Input: part model. Units: mm. Frame: model coordinates. Face numbers are marked on the shaded views. A direction names the side the tool comes from. Coordinates: 2 decimals unless noted, no trailing zeros. Loops run counter-clockwise (first coordinate to the right, second up) from the corner with the lowest first, then second, coordinate; pieces in that order, holes last.
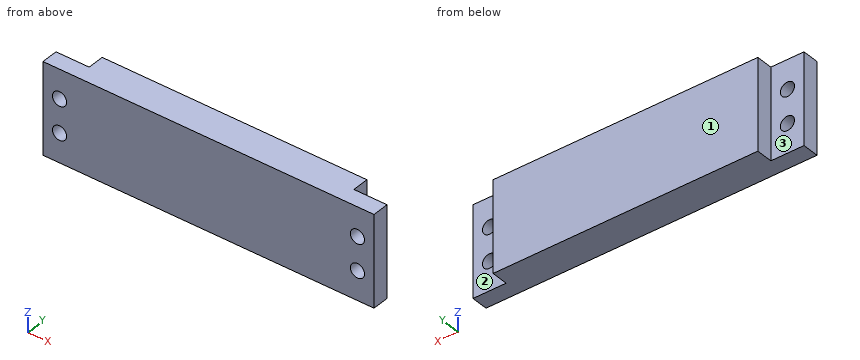
```python
from build123d import *

# Parameters (mm, degrees)
SKETCH1_W           = 63.5
SKETCH1_H           = 17.4625
BOSS_EXTRUDE1_DEPTH = 6.35
SKETCH2_W           = 6.35
SKETCH2_H           = 3.175
CUT_EXTRUDE1_DEPTH  = 67.1627645
SKETCH3_R           = 1.357929869
CUT_EXTRUDE2_DEPTH  = 67.1627645


with BuildPart() as part:
    # Sketch1 → Boss-Extrude1 (new body)
    with BuildSketch(Plane(origin=(0, 0, 0), x_dir=(1, 0, 0), z_dir=(0, 1, 0))):
        with Locations((-31.75, 8.73125)):
            Rectangle(SKETCH1_W, SKETCH1_H)
    extrude(amount=BOSS_EXTRUDE1_DEPTH)

    # Sketch2 → Cut-Extrude1 (cut, through all)
    with BuildSketch(Plane.XY):
        with Locations((-3.175, 4.7625)):
            Rectangle(SKETCH2_W, SKETCH2_H)
        with Locations((-60.325, 4.7625)):
            Rectangle(SKETCH2_W, SKETCH2_H)
    extrude(amount=-CUT_EXTRUDE1_DEPTH, mode=Mode.SUBTRACT)

    # Sketch3 → Cut-Extrude2 (cut, through all)
    with BuildSketch(Plane(origin=(0, 6.35, 0), x_dir=(1, 0, 0), z_dir=(0, 1, 0))):
        with Locations(Location((-60.325, 11.90625, 0), (0, 0, 270))):
            Circle(SKETCH3_R)
        with Locations(Location((-60.325, 5.55625, 0), (0, 0, 90))):
            Circle(SKETCH3_R)
        with Locations(Location((-3.175, 5.55625, 0), (0, 0, 270))):
            Circle(SKETCH3_R)
        with Locations(Location((-3.175, 11.90625, 0), (0, 0, 90))):
            Circle(SKETCH3_R)
    extrude(amount=-CUT_EXTRUDE2_DEPTH, mode=Mode.SUBTRACT)


solid = part.part
```
Item 1: Line query: L1, parallel to X at y = 0.5, z = -12; L2, parallel to X at y = 3, z = -11.5; L3, parallel to Y at x = -3.5, z = -3 (3 decimals). Output: solid intervals per line, ascending.
Result:
L1: x = -63.5 to -61.68, -58.97 to -4.53, -1.82 to 0
L2: x = -63.5 to -61.62, -59.03 to -4.47, -1.88 to 0
L3: y = 0 to 3.175
Item 2: Section query A-A (z = -5.5). Output: boundary loops of the cut face in (x, y) (3 decimals), then the cut area to 3 significant figures.
Result:
outline: (-63.5, 0) - (-61.682, 0) - (-61.682, 3.175) - (-63.5, 3.175) - close; (-58.968, 0) - (-4.532, 0) - (-4.532, 3.175) - (-6.35, 3.175) - (-6.35, 6.35) - (-57.15, 6.35) - (-57.15, 3.175) - (-58.968, 3.175) - close; (-1.818, 0) - (0, 0) - (0, 3.175) - (-1.818, 3.175) - close
area: 346 mm2
Item 3: Section query C-C (y = 1.25). Output: boundary loops of the cut face in (x, z) (1 decimal).
Result:
outline: (-63.5, -17.5) - (0, -17.5) - (0, 0) - (-63.5, 0) - close; hole circle Ø2.7 at (-60.3, -11.9); hole circle Ø2.7 at (-60.3, -5.6); hole circle Ø2.7 at (-3.2, -11.9); hole circle Ø2.7 at (-3.2, -5.6)
Item 4: Section query B-B (z = -14.5). Output: boundary loops of the cut face in (x, y) (3 decimals), then the cut area to 3 significant figures.
Result:
outline: (-63.5, 0) - (0, 0) - (0, 3.175) - (-6.35, 3.175) - (-6.35, 6.35) - (-57.15, 6.35) - (-57.15, 3.175) - (-63.5, 3.175) - close
area: 363 mm2
Item 5: Contact query for flat-ended pins moving along their axis: P1, Ø3, axis at x = -60.32, z = -5.56, coming from the +Y side (3 decimals); P2, Ø4, axis at x = -53, z = -15, coming from the -Y side; P3, Ø2.5, axis at y = 5.5, z = -6, coming from the -X side; P4, Ø2, axis at y = 5.5, z = -4.5, coming from the +X side. Output: stop coordinate, or through.
Result:
P1: stops at y = 3.175
P2: stops at y = 0
P3: stops at x = -57.15
P4: stops at x = -6.35
Item 6: Section query D-D (y = 5). Output: boundary loops of the cut face in (x, z).
Result:
outline: (-57.15, -17.46) - (-6.35, -17.46) - (-6.35, 0) - (-57.15, 0) - close
Item 7: Reachability of the marked faces 1, 2 and 3 from +Z, -Z, +X, -X, +Y, -Y: full face, straight path, thin tool, end or side. Return the list, or none.
Result:
face 1: +Z, -Z, +X, -X, +Y
face 2: +Z, -Z, +X, +Y
face 3: +Z, -Z, -X, +Y
